Can you work these out from the drawing? Everything is in mm from the part's minimum corner. Round coordinates to 2 decimals unless told otherwise and drop trailing zeros. Order: outer loops, then holes, each group sorted by start corner. A loop starts at its lowest first (then second) coordinate and runs counter-clockwise, first axis right, second up. Notation, with made-up numbers: (34.5, -38.75) -> (73.5, -38.75) arc R17 ccw to (73.5, -29.75) -> close; hole circle Ø8 at (-28.75, 71.5). An arc over 180 degrees is marked (long way). One line per item, written item: value.
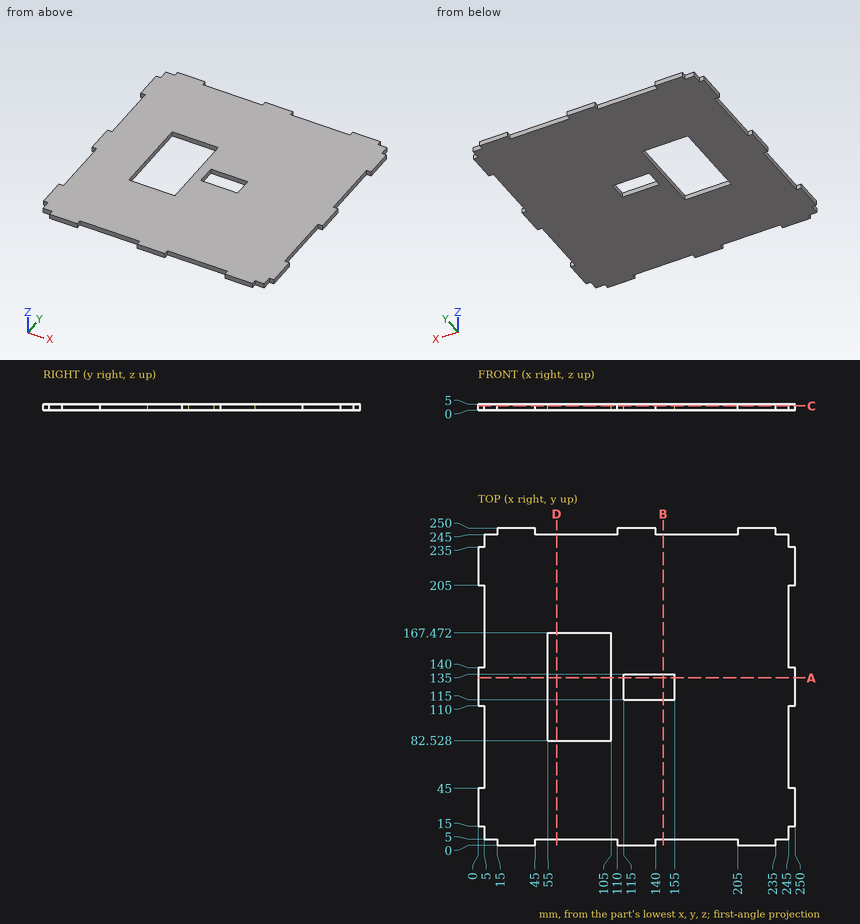
Q1. For P1, Ø1.5, axis at x = 247.5, z = 1.5, coming from the -Y side; P2, Ø1.5, axis at y = 2.5, z = 3.5, coming from the -X side; P3, Ø2.5, axis at y = 11.5, z = 3, coming from the +X side, each with a flat end and sliding along its axis, tell me the tip position at first contact or that it passes through.
Answers:
P1: y = 15
P2: x = 15
P3: x = 245
Q2. I want a section at B-B on x = 146. Write out the boundary of the cut face in (y, z).
Answers:
outline: (5, 0) -> (115, 0) -> (115, 5) -> (5, 5) -> close; (135, 0) -> (245, 0) -> (245, 5) -> (135, 5) -> close
Q3. I want a section at A-A on y = 132. Write out the boundary of the cut face in (x, z).
Answers:
outline: (0, 0) -> (55, 0) -> (55, 5) -> (0, 5) -> close; (105, 0) -> (115, 0) -> (115, 5) -> (105, 5) -> close; (155, 0) -> (250, 0) -> (250, 5) -> (155, 5) -> close
Q4. I want a section at D-D on x = 62. Write out the boundary of the cut face in (y, z), then the cut area to 3 significant figures.
Answers:
outline: (5, 0) -> (82.53, 0) -> (82.53, 5) -> (5, 5) -> close; (167.47, 0) -> (245, 0) -> (245, 5) -> (167.47, 5) -> close
area: 775 mm2
Q5. I need wall thicknesses on line 1 along X through (y, z) = (120.5, 1.7); line 2 along X through (y, z) = (99, 2.05); line 3 along Y through (x, z) = (116, 4.35). Which ranges of each line are inside material? Lowest first, please.
Answers:
line 1: 0 to 55, 105 to 115, 155 to 250
line 2: 5 to 55, 105 to 245
line 3: 0 to 115, 135 to 250
Q6. I want a section at C-C on z = 3.55. Give the number of separate pieces and of enclosed holes in the cut face, then the cut area to 3 significant figures.
Answers:
separate pieces: 1
enclosed holes: 2
area: 54,400 mm2
